```python
from build123d import *

# Parameters (mm, degrees)
F1_DEPTH    = 101.6
F2_R        = 25.4
F3_R        = 76.2
F4_R        = 25.4
F5_T1_DEPTH = 101.6
F6_R        = 44.7643478735
F7_R        = 304.8


# Not quite as in the source:
# - a fillet or chamfer that OpenCascade refuses, or shapes differently, is made with other operations: its cross-section is extruded or revolved along the edge and cut away or added


with BuildPart() as f1:
    # F0 (on Front) → F1 (new body)
    with BuildSketch(Plane.XZ):
        Polygon((228.6, -76.2), (228.6, 76.2), (-228.6, 76.2), (-228.6, 29.4590149546), (-86.9704671455, -76.2), align=None)
        Polygon((-50.8129218496, -47.2383520842), (-177.8, 29.4590149546), (-177.8, 54.8590149546), (194.0227749825, 54.8590149546), (194.0227749825, -47.2383520842), align=None, mode=Mode.SUBTRACT)
    extrude(amount=F1_DEPTH)

    # F2
    f2_edges = [f1.edges().sort_by_distance(p)[0] for p in [
        (-228.6, -50.8, 76.2),
        (-228.6, -50.8, 29.459015),
    ]]
    fillet(f2_edges, radius=F2_R)

    # F3
    f3_edges = [f1.edges().sort_by_distance(p)[0] for p in [
        (-86.970467, -50.8, -76.2),
        (228.6, -50.8, -76.2),
    ]]
    fillet(f3_edges, radius=F3_R)

    # F4
    f4_edges = [f1.edges().sort_by_distance(p)[0] for p in [
        (228.6, -50.8, 76.2),
    ]]
    fillet(f4_edges, radius=F4_R)

    # F5: fillet of radius 17.78 on 2 edges, made by hand

    # F5_s2 → F5_t1 (join)
    with BuildSketch(Plane.XZ):
        with BuildLine():
            ThreePointArc((-169.2122093999, 24.2721806932), (-175.5049262693, 30.7540427919), (-177.8, 39.4916316146))
            Line((-177.8, 39.4916316146), (-177.8, 29.4590149546))
            Line((-177.8, 29.4590149546), (-169.2122093999, 24.2721806932))
        make_face()
        with BuildLine():
            ThreePointArc((-177.8, 37.0790149546), (-172.5923585695, 49.6513735241), (-160.02, 54.8590149546))
            Line((-160.02, 54.8590149546), (-177.8, 54.8590149546))
            Line((-177.8, 54.8590149546), (-177.8, 37.0790149546))
        make_face()
    extrude(amount=F5_T1_DEPTH)

    # F6
    f6_edges = [f1.edges().sort_by_distance(p)[0] for p in [
        (194.022775, -50.8, -47.238352),
        (194.022775, -50.8, 54.859015),
    ]]
    fillet(f6_edges, radius=F6_R)

    # F7
    f7_edges = [f1.edges().sort_by_distance(p)[0] for p in [
        (-50.812922, -50.8, -47.238352),
    ]]
    fillet(f7_edges, radius=F7_R)


solid = f1.part
```
For this review, take the finished solid that the model builds, in its own axes (mm). A direction names the side the tool comes from. Round coordinates to 2 decimals unless told otherwise and drop trailing zeros. Write each loop counter-clockwise with the first axis right and the second up, starting at its lowest first coordinate (ties: lowest second). Pieces come first, ordered by that corner, then holes. Notation, with made-up numbers: (-30, 60.5) - (-6, 60.5) arc R34 cw to (-6, 96.5) - close; hole circle Ø5 at (15, -33). An arc over 180 degrees is marked (long way). Answer as CSV lines item,"result". Start each with the question number.
(1) Add section B-B, the plane y = -8.5. State the section outline as (x, z) points, plus the area to 3 significant figures.
(2) Add section A-A, the plane x = 133. State the section outline as (y, z) points, plus the area to 3 significant figures.
(3) Machinability: for faces 4 (the flat face through (228.6, -50, 25)), 5 (the flat face through (92, -50, -47.238)), which of the approach directions +Z, -Z, +X, -X, +Y, -Y give a long, thin tool a straight path to every point of the face, cutting with its end or side? Answer none if there is none.
(4) Mouldability with a two-part tool opening along Z and no side actions: class faces 1 (the flat face through (-163.59, -50.09, -19.04)), 2 (the cylindrical face through (-175.137, -50.089, 30.132)), 3 (the flat face through (3, -50, 76.2)) as +Z half, -Z half, draft (parallel to the pull), parting line (faces both ways), or undercut.
(5) For pin 1 (5 mm diameter, centred on y = -12.5, z = -59, fed in from +X); pin 2 (10 mm diameter, centred on y = -12.5, z = -24.5, fed in from -X); pin 3 (1.5 mm diameter, centred on y = -33.5, z = -37.5, fed in from +X), all flat-tipped, find the tip position at first contact; note any pin that passes through.
(6) Add section D-D, the plane z = -53.5. State the section outline as (x, y) points, plus the area to 3 significant figures.
(7) For line 1 (Z direction, x = 112.5, y = -82.5); line 2 (X direction, y = -23.5, z = -11.5); line 3 (Z direction, x = -50.5, y = -77), list the stretches that pass through material, from the lowest coordinate up.
(8) Add section C-C, the plane z = -17.5. State the section outline as (x, y) points, plus the area to 3 significant figures.
From the geometry:
1,outline,"(-228.6, 42.2) arc R25.4 ccw to (-218.39, 21.84) - (-107.24, -61.08) arc R76.2 ccw to (-61.68, -76.2) - (152.4, -76.2) arc R76.2 ccw to (228.6, 0) - (228.6, 50.8) arc R25.4 ccw to (203.2, 76.2) - (-203.2, 76.2) arc R25.4 ccw to (-228.6, 50.8) - close; hole (-177.76, 38.29) arc R17.78 ccw to (-169.21, 24.27) - (-123.49, -3.34) arc R304.8 ccw to (34.09, -47.24) - (149.26, -47.24) arc R44.76 ccw to (194.02, -2.47) - (194.02, 10.09) arc R44.76 ccw to (149.26, 54.86) - (-160.02, 54.86) arc R17.78 ccw to start"
1,area,"29,100 mm²"
2,outline,"(-101.6, -76.2) - (0, -76.2) - (0, -47.24) - (-101.6, -47.24) - close; (-101.6, 54.86) - (0, 54.86) - (0, 76.2) - (-101.6, 76.2) - close"
2,area,"5,110 mm²"
3,face 4,"+Z, -Z, +X, +Y, -Y"
3,face 5,"+Y, -Y"
4,face 1,"-Z half"
4,face 2,"undercut"
4,face 3,"+Z half"
5,pin 1,"stops at x = 203.53"
5,pin 2,"stops at x = -162.97"
5,pin 3,"stops at x = 219.15"
6,outline,"(-117.4, -101.6) - (206.66, -101.6) - (206.66, 0) - (-117.4, 0) - close"
6,area,"32,900 mm²"
7,line 1,"z = -76.2 to -47.24, 54.86 to 76.2"
7,line 2,"x = -173.7 to -109.12, 193.1 to 227.73"
7,line 3,"z = -76.2 to -35.26, 54.86 to 76.2"
8,outline,"(-165.65, -101.6) - (-97.23, -101.6) - (-97.23, 0) - (-165.65, 0) - close; (191.43, -101.6) - (226.56, -101.6) - (226.56, 0) - (191.43, 0) - close"
8,area,"10,500 mm²"
